```python
from build123d import *

# Parameters (mm, degrees)
F0_W     = 107.95
F0_H     = 57.15
F0_W_2   = 5.6642
F0_H_2   = 0.17526
F1_DEPTH = 12.7


with BuildPart() as f1:
    # F0 (on Front) → F1 (new body)
    with BuildSketch(Plane.XZ):
        Rectangle(F0_W, F0_H)
        Polygon((50.8, -5.9944), (50.8, -25.4), (27.5717, -25.4), (26.8224, -25.4), (11.9888, -25.4), (10.02665, -25.4), (-50.8, -25.4), (-50.8, 25.4), (10.02665, 25.4), (11.9888, 25.4), (50.8, 25.4), (50.8, -4.78282), align=None, mode=Mode.SUBTRACT)
        Polygon((10.02665, -25.4), (11.9888, -25.4), (11.9888, -15.017242), (11.9888, -14.5542), (11.9888, -5.9944), (11.9888, -4.78282), (11.9888, 25.4), (10.02665, 25.4), align=None)
        Polygon((27.5717, -5.9944), (50.8, -5.9944), (50.8, -4.78282), (11.9888, -4.78282), (11.9888, -5.9944), (20.872196, -5.9944), (21.1582, -5.9944), (26.8224, -5.9944), align=None)
        Polygon((26.8224, -25.4), (27.5717, -25.4), (27.5717, -5.9944), (26.8224, -5.9944), (26.8224, -11.53414), (26.8224, -11.7094), (26.8224, -14.5542), (26.8224, -15.017242), align=None)
        Polygon((11.9888, -15.017242), (26.8224, -15.017242), (26.8224, -14.5542), (21.1582, -14.5542), (20.872196, -14.5542), (19.4056, -14.5542), (11.9888, -14.5542), align=None)
        Polygon((21.1582, -11.53414), (21.1582, -5.9944), (20.872196, -5.9944), (20.872196, -14.5542), (21.1582, -14.5542), (21.1582, -11.7094), align=None)
        with Locations((23.9903, -11.62177)):
            Rectangle(F0_W_2, F0_H_2)
    extrude(amount=F1_DEPTH)


solid = f1.part
```
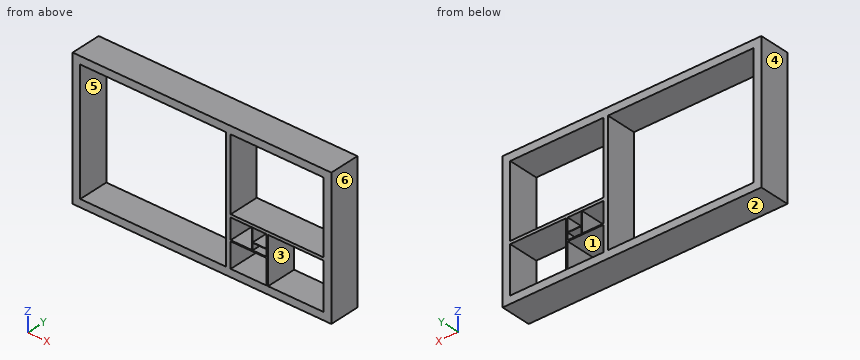
The listing builds one solid part. Answer for the finished solid, in the listing's coordinates (mm). Face numbers are marked on the shaded views. A direction names the side the tool comes from. Give positions to 0.01 mm unless a question says otherwise; leave off trailing zeros. Order: outer loops, then holes, each group sorted by start corner. A loop starts at its lowest first (then second) coordinate and runs counter-clockwise, first axis right, second up.
1) Find section B-B on z = -7. Write down the section's boundary in (x, y) (3 decimals), then the cut area to 3 significant figures.
Reported:
outline: (-53.975, -12.7) - (-50.8, -12.7) - (-50.8, 0) - (-53.975, 0) - close; (10.027, -12.7) - (11.989, -12.7) - (11.989, 0) - (10.027, 0) - close; (20.872, -12.7) - (21.158, -12.7) - (21.158, 0) - (20.872, 0) - close; (26.822, -12.7) - (27.572, -12.7) - (27.572, 0) - (26.822, 0) - close; (50.8, -12.7) - (53.975, -12.7) - (53.975, 0) - (50.8, 0) - close
area: 119 mm2
2) Find section C-C on x = -42. Write down the section's boundary in (y, z) (3 decimals).
Reported:
outline: (-12.7, -28.575) - (0, -28.575) - (0, -25.4) - (-12.7, -25.4) - close; (-12.7, 25.4) - (0, 25.4) - (0, 28.575) - (-12.7, 28.575) - close
3) For the marked faces 5 and 6, determine the directions among +Z, -Z, +X, -X, +Y, -Y from which every point of the face is accessible in a straight line to the end or side of a thin tool.
Reported:
face 5: +Y, -Y
face 6: +Z, -Z, +X, +Y, -Y
4) Find section A-A on x = 42.5. Write down the section's boundary in (y, z) (3 decimals).
Reported:
outline: (-12.7, -28.575) - (0, -28.575) - (0, -25.4) - (-12.7, -25.4) - close; (-12.7, -5.994) - (0, -5.994) - (0, -4.783) - (-12.7, -4.783) - close; (-12.7, 25.4) - (0, 25.4) - (0, 28.575) - (-12.7, 28.575) - close
5) Consider line 1 along Z through (x, y) = (22.5, -10) (3 decimals); line 2 along Z through (x, y) = (28, -11) (3 decimals); line 3 along X through (y, z) = (-8.5, 10) (3 decimals). Determine where each line is inside the solid, lowest interval first.
Reported:
line 1: z = -28.575 to -25.4, -15.017 to -14.554, -11.709 to -11.534, -5.994 to -4.783, 25.4 to 28.575
line 2: z = -28.575 to -25.4, -5.994 to -4.783, 25.4 to 28.575
line 3: x = -53.975 to -50.8, 10.027 to 11.989, 50.8 to 53.975
6) Find section D-D on y = -9.25. Give the number of separate pieces and of enclosed holes in the cut face, then the cut area to 3 significant figures.
Reported:
separate pieces: 1
enclosed holes: 7
area: 1,180 mm2
7) Determine the mould class of the marked faces 1, 2, 3 and 4 for opening direction Z: pulls with the +Z half, pulls with the -Z half, needs draft (parallel to the pull), parting line crosses it, or undercut.
Reported:
face 1: undercut
face 2: pulls with the -Z half
face 3: undercut
face 4: needs draft
